Study the drawing (mm; zero at the part's minimum x, y, z) and answer. A direction names the side the tool comes from. Coordinates: 2 decimals unless noted, no trailing zeros. Write each loop counter-clockwise with the first axis right and the second up, starting at its lowest first coordinate (ties: lowest second). Pieces come first, ordered by that corner, then holes. Notation, with made-up numbers: M 30.25,-11.75 L 53.25,-11.75 A20 cw 53.25,20.25 Z; hole C 68.5,76 d5. An arc over 180 degrees is marked long. Answer as a JSON object with one key per item and string values. Group by question number.
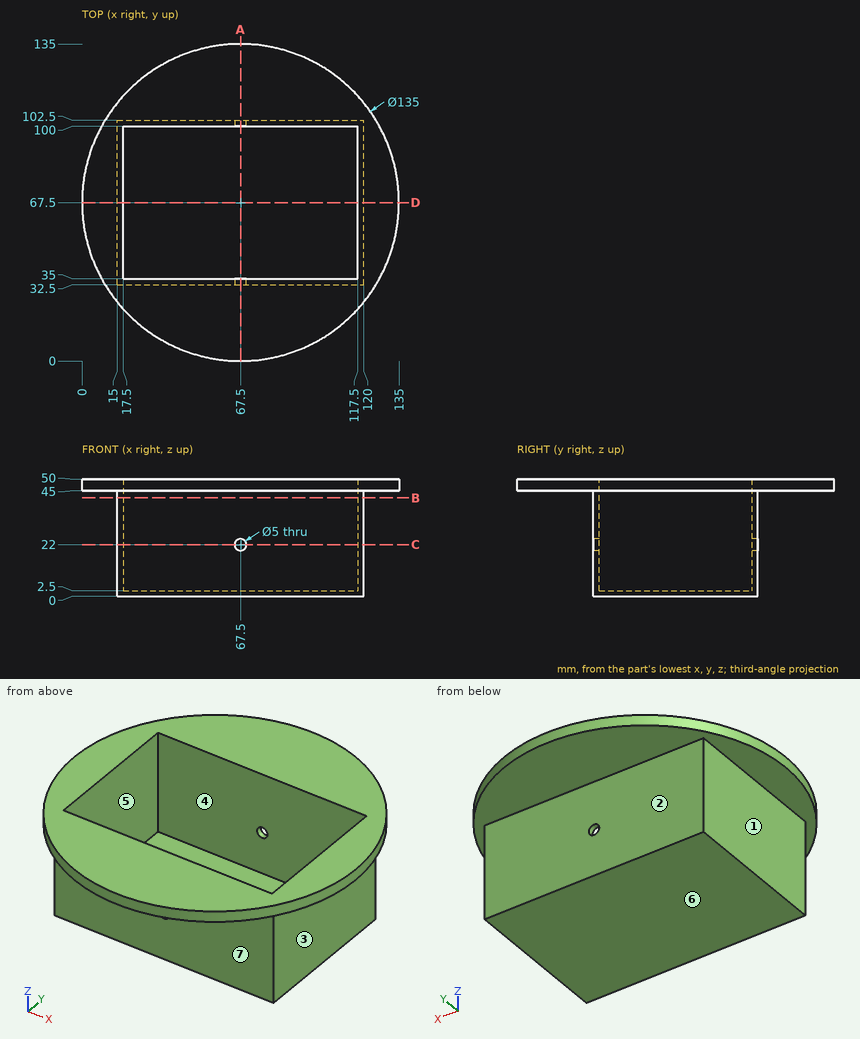
Item 1: A cutting plane is placed at A-A, the plane x = 67.5. Write down the section's boundary in (y, z).
Item 2: A cutting plane is placed at D-D, the plane y = 67.5. Write down the section's boundary in (x, z), and give its area (3 significant figures).
Item 3: Consider L1, parallel to Y at x = 91.5, z = 8; L2, parallel to X at y = 56, z = 43.5; L3, parallel to Z at x = 67.5, y = 33.1. Determine where each line is inside the solid, lowest interval first. Write a range as from..to.
Item 4: A cutting plane is placed at C-C, the plane z = 22. Write down the section's boundary in (x, y), and give its area (3 significant figures).
Item 5: For a pull along Y with two mould halves and no side action, classify the marked faces 4, 5, 6 and 7 as +Y half, -Y half, draft (parallel to the pull), parting line (faces both ways), or undercut.
Item 6: A tool of negligible diameter and unlimited length cuts with its end or side. For the marked faces 1, 2 and 3, from which of +Z, -Z, +X, -X, +Y, -Y can it reach the whole face along a straight path? Write none if from no direction.
Item 7: A cutting plane is placed at B-B, the plane z = 42. Write down the section's boundary in (x, y).
Item 8: Flat-ended cylindrical pins translate along their axes: pin 1 Ø12 at (x, z) = (101.5, 14) entering from +Y; pin 2 Ø13.5 at (y, z) = (69.5, 28) entering from +X; pin 3 Ø6 at (x, y) = (53.5, 93) entering from +Z; pin 4 Ø4.5 at (x, z) = (67.5, 22) entering from +Y. Find the tip coordinate at first contact, or state that the pin passes through.
Answer:
{
 "1": {"outline": "M 0,45 L 32.5,45 L 32.5,24.5 L 35,24.5 L 35,50 L 0,50 Z; M 32.5,0 L 102.5,0 L 102.5,19.5 L 100,19.5 L 100,2.5 L 35,2.5 L 35,19.5 L 32.5,19.5 Z; M 100,24.5 L 102.5,24.5 L 102.5,45 L 135,45 L 135,50 L 100,50 Z"},
 "2": {"outline": "M 0,45 L 15,45 L 15,0 L 120,0 L 120,45 L 135,45 L 135,50 L 117.5,50 L 117.5,2.5 L 17.5,2.5 L 17.5,50 L 0,50 Z", "area": "650 mm2"},
 "3": {"L1": "32.5..35, 100..102.5", "L2": "15..17.5, 117.5..120", "L3": "0..19.5, 24.5..50"},
 "4": {"outline": "M 15,32.5 L 65,32.5 L 65,35 L 17.5,35 L 17.5,100 L 65,100 L 65,102.5 L 15,102.5 Z; M 70,32.5 L 120,32.5 L 120,102.5 L 70,102.5 L 70,100 L 117.5,100 L 117.5,35 L 70,35 Z", "area": "825 mm2"},
 "5": {"face 4": "undercut", "face 5": "undercut", "face 6": "draft", "face 7": "-Y half"},
 "6": {"face 1": "-Z, -X, +Y, -Y", "face 2": "-Z, +X, -X, +Y", "face 3": "-Z, +X, +Y, -Y"},
 "7": {"outline": "M 15,32.5 L 120,32.5 L 120,102.5 L 15,102.5 Z; hole M 17.5,35 L 117.5,35 L 117.5,100 L 17.5,100 Z"},
 "8": {"pin 1": "y = 102.5", "pin 2": "x = 120", "pin 3": "z = 2.5", "pin 4": "through"}
}
